Part model, mm, in its own coordinate system. A direction names the side the tool comes from. Round coordinates to 2 decimals unless told otherwise and drop trailing zeros. Order: outer loops, then holes, each group sorted by start corner. A loop starts at its lowest first (then second) coordinate and runs counter-clockwise, first axis right, second up. Notation, with made-up numbers: M 48,88 L 84,88 A16 ccw 84,93 Z; hole C 14.5,87.5 d6. An arc over 180 degrees is marked long. Write each question's results on one line, items separated by ' | '. Start each with the question number.
1. Band-saw the part on C-C, the plane y = -27. List the corners of the cut face in (x, z), then the cut area to 3 significant figures.
2. Band-saw the part on B-B, the plane z = 0.65. List the corners of the cut face in (x, y).
3. Two-plate mould, pull along X, no slides. Class faces 1 (the face through (-15, -21, 2)), 2 (the face through (-19, -10, 1)), 3 (the face through (-12.1, -9.28, 1.52)): +X half, -X half, draft (parallel to the pull), parting line (faces both ways), or undercut.
4. Band-saw the part on A-A, the plane x = 14. List the corners of the cut face in (y, z).
5. Which spindle directions (+Z, -Z, +X, -X, +Y, -Y) get a long thin tool onto all of the face, cutting with end or side? Do faces 4 (the face through (-14.8, -39, 1)), 5 (the face through (-13, -33, 2)), 6 (the face through (0, -20, 0)). Say none if no direction does.
6. Drop flat-ended pins along their axis: pin 1 Ø0.8 at (x, z) = (-13, 2) entering from +Y; pin 2 Ø1.5 at (x, z) = (1.5, 1) entering from +Y; pin 3 Ø10 at (x, y) = (-8, 1.5) entering from -Z. Give the stop position or say it passes through.
7. Band-saw the part on D-D, the plane x = 0. List the corners of the cut face in (y, z).
8. Probe L1, parallel to Y at x = 0, z = 2.2; L2, parallel to Y at x = -9.5, z = 1.3; L3, parallel to Y at x = -12.5, z = 0.7. List the from-to ranges inside material, lowest first. Write a range as [from, to].
```python
from build123d import *

# Parameters (mm, degrees)
SKETCH1_R           = 2.5
SKETCH1_R_2         = 1.5
BOSS_EXTRUDE1_DEPTH = 3
SKETCH2_R           = 15.25
SKETCH2_R_2         = 3
CUT_EXTRUDE1_DEPTH  = 49.938737213


with BuildPart() as part:
    # Sketch1 → Boss-Extrude1 (new body)
    with BuildSketch(Plane.XY):
        with BuildLine():
            Line((-19, 0), (-19, -32))
            Line((-19, -32), (-14.8, -32))
            Line((-14.8, -32), (-14.8, -45))
            Line((-14.8, -45), (19, -45))
            Line((19, -45), (19, 0))
            ThreePointArc((19, 0), (0, 19), (-19, 0))
        make_face()
        Circle(SKETCH1_R, mode=Mode.SUBTRACT)
        with Locations((-14, -27)):
            Circle(SKETCH1_R_2, mode=Mode.SUBTRACT)
        with Locations(Location((14, -27, 0), (0, 0, 180))):
            Circle(SKETCH1_R_2, mode=Mode.SUBTRACT)
    extrude(amount=BOSS_EXTRUDE1_DEPTH)

    # Sketch2 → Cut-Extrude1 (cut, through all)
    with BuildSketch(Plane.XY.offset(3)):
        Circle(SKETCH2_R)
        with Locations((14, -27)):
            Circle(SKETCH2_R_2)
        with BuildLine():
            Line((-12, -21), (-19, -21))
            Line((-19, -21), (-19, -32))
            Line((-19, -32), (-14.8, -32))
            Line((-14.8, -32), (-14.8, -33))
            Line((-14.8, -33), (-12, -33))
            ThreePointArc((-12, -33), (-6, -27), (-12, -21))
        make_face()
    extrude(amount=-CUT_EXTRUDE1_DEPTH, mode=Mode.SUBTRACT)


solid = part.part
```
Solution:
1) outline: M -6,0 L 11,0 L 11,3 L -6,3 Z; M 17,0 L 19,0 L 19,3 L 17,3 Z | area: 57.0 mm^2
2) outline: M -19,-21 L -12,-21 A6 cw -12,-33 L -14.8,-33 L -14.8,-45 L 19,-45 L 19,0 A19 ccw -19,0 Z; hole C 0,0 d30.5; hole C 14,-27 d6
3) face 1: draft | face 2: -X half | face 3: undercut
4) outline: M -45,0 L -30,0 L -30,3 L -45,3 Z; M -24,0 L -6.05,0 L -6.05,3 L -24,3 Z; M 6.05,0 L 12.85,0 L 12.85,3 L 6.05,3 Z
5) face 4: +Z, -Z, -X, -Y | face 5: +Z, -Z, -X | face 6: -Z, +X, -X, +Y, -Y
6) pin 1: y = 14.22 | pin 2: y = 18.99 | pin 3: through
7) outline: M -45,0 L -15.25,0 L -15.25,3 L -45,3 Z; M 15.25,0 L 19,0 L 19,3 L 15.25,3 Z
8) L1: [-45, -15.25], [15.25, 19] | L2: [-45, -32.45], [-21.55, -11.93], [11.93, 16.45] | L3: [-45, -33], [-21, -8.74], [8.74, 14.31]
